Work out the finished part from the listing and answer in its coordinate system (mm). Give positions to 0.01 mm unless a question says otherwise; leave off trailing zeros. Write each loop counter-clockwise with the first axis right and the second up, starting at its lowest first coordinate (ties: lowest second). Pieces come first, ordered by that corner, then holes.
1) Find section C-C (x = 29). Determine the outline of the cut face in (y, z), plus the area to 3 significant figures.
2) Find section A-A (z = 0.2). Determine the outline of the cut face in (x, y), plus the area to 3 significant figures.
3) Straight lines are drawn through the part: probe 1 along Y at (x, z) = (3.5, 0.1); probe 2 along Y at (x, z) = (0.5, 0.15); probe 3 along Y at (x, z) = (18, 0.3). For each, find the intervals that lie inside material, in ascending order.
4) Find section D-D (y = 7.5). Determine the outline of the cut face in (x, z), plus the area to 3 significant figures.
5) Find section B-B (y = 6). Determine the outline of the cut face in (x, z), plus the area to 3 significant figures.
```python
from build123d import *

# Parameters (mm, degrees)
PAD_DEPTH = 0.5


with BuildPart() as part:
    # Sketch → Pad (new body)
    with BuildSketch(Plane.XY):
        Polygon((-3.256772, 2.764826), (-3.256772, 8.764826), (6.743228, 8.764826), (10.243228, 9.764826), (35.243228, 9.764826), (15.243228, 1.764826), (10.243228, 1.764826), (6.743228, 2.764826), align=None)
        with BuildLine():
            ThreePointArc((2.243228, 7.014826), (0.993228, 5.764826), (2.243228, 4.514826))
            Line((2.243228, 4.514826), (4.743228, 4.514826))
            ThreePointArc((4.743228, 4.514826), (5.993228, 5.764826), (4.743228, 7.014826))
            Line((2.243228, 7.014826), (4.743228, 7.014826))
        make_face(mode=Mode.SUBTRACT)
    extrude(amount=PAD_DEPTH)


solid = part.part
```
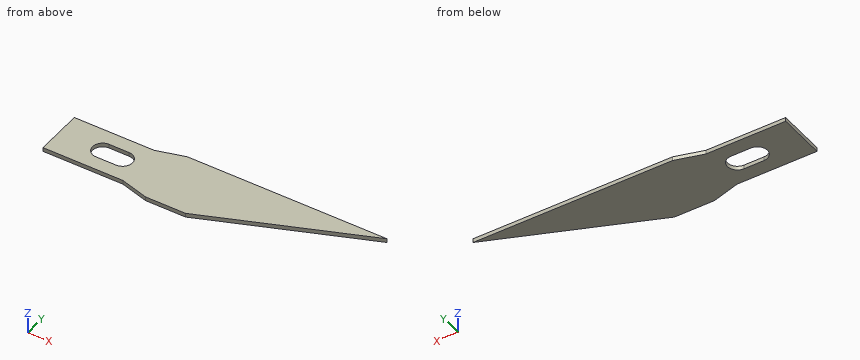
Results:
1. outline: (7.27, 0) - (9.76, 0) - (9.76, 0.5) - (7.27, 0.5) - close
1. area: 1.25 mm2
2. outline: (-3.26, 2.76) - (6.74, 2.76) - (10.24, 1.76) - (15.24, 1.76) - (35.24, 9.76) - (10.24, 9.76) - (6.74, 8.76) - (-3.26, 8.76) - close; hole (2.24, 4.51) - (4.74, 4.51) arc R1.25 ccw to (4.74, 7.01) - (2.24, 7.01) arc R1.25 ccw to start
2. area: 193 mm2
3. probe 1: y = 2.76 to 4.51, 7.01 to 8.76
3. probe 2: y = 2.76 to 8.76
3. probe 3: y = 2.87 to 9.76
4. outline: (-3.26, 0) - (29.58, 0) - (29.58, 0.5) - (-3.26, 0.5) - close
4. area: 16.4 mm2
5. outline: (-3.26, 0) - (1.02, 0) - (1.02, 0.5) - (-3.26, 0.5) - close; (5.97, 0) - (25.83, 0) - (25.83, 0.5) - (5.97, 0.5) - close
5. area: 12.1 mm2
